CAD build for the part. Positions are in the model's coordinates, mm. Face numbers are marked on the shaded views. Round coordinates to 2 decimals unless told otherwise and drop trailing zeros. Order: outer loops, then holes, each group sorted by start corner. A loop starts at its lowest first (then second) coordinate and runs counter-clockwise, first axis right, second up. Notation, with made-up numbers: M -15,11 L 17,11 A17 ccw 17,38 Z; hole C 33,4 d3. An arc over 180 degrees is marked long. Put each result on its own line as item: value.
Autodesk Inventor part; units mm, degrees
ref_plane "YZ Plane" through (0, 0, 0) normal (1, 0, 0) x (0, 1, 0)
ref_plane "XZ Plane" through (0, 0, 0) normal (0, 1, 0) x (-1, 0, 0)
ref_plane "XY Plane" through (0, 0, 0) normal (0, 0, 1) x (1, 0, 0)
sketch "Sketch1" plane through (0, 0, 0) normal (0, 1, 0) x (-1, 0, 0)
  line L0 (0, 0) -> (0, -60) construction
  line L1 (-60, 0) -> (-60, -60)
  line L2 (60, -60) -> (60, 0)
  arc A0 (60, 0) -> (-60, 0) centre (0, 0) ccw
  arc A1 (-60, -60) -> (60, -60) centre (0, -60) ccw
  line L3 (56, 0) -> (56, -60)
  arc A2 (-56, -60) -> (56, -60) centre (0, -60) ccw
  line L4 (-56, -60) -> (-56, 0)
  arc A3 (56, 0) -> (-56, 0) centre (0, 0) ccw
  point P0 (0, -30)
  dimension "d0" = 60
  dimension "d1" = 60
  dimension "d4" = 4
extrude "Extrusion2" add sketch "Sketch1" along normal blind 70
extrude "Extrusion3" add sketch "Sketch1" along normal blind 4 contours L3 A2 L4 A3
fillet "Fillet1" radius 50.8 8 edges at (0, 4, 56) (-56, 4, -30) (0, 4, -116) (56, 4, -30) (0, 0, 60) (60, 0, -30) (0, 0, -120) (-60, 0, -30)
sketch "Sketch5" plane through (0, 70, 0) normal (0, 1, 0) x (1, 0, 0)
  line L0 (-9, 118.645) -> (9, 118.645)
  line L1 (9, 118.645) -> (9, -58.355)
  line L2 (9, -58.355) -> (-9, -58.355)
  line L3 (-9, -58.355) -> (-9, 118.645)
  point P0 (0, 0)
  dimension "d11" = 177
  dimension "d12" = 18
  dimension "d13" = 9
extrude "Extrusion4" add sketch "Sketch5" against normal blind 10
extrude "Extrusion5" cut sketch "Sketch5" against normal blind 9
sketch "Sketch6" plane through (0, 61, 0) normal (0, 1, 0) x (1, 0, 0)
  line L0 (-9, 118.6362) -> (9, 118.6362)
  line L1 (9, 118.6362) -> (9, -58.3638)
  line L2 (9, -58.3638) -> (-9, -58.3638)
  line L3 (-9, -58.3638) -> (-9, 118.6362)
  line L4 (-8, 117.6362) -> (8, 117.6362)
  line L5 (8, 117.6362) -> (8, -57.3638)
  line L6 (8, -57.3638) -> (-8, -57.3638)
  line L7 (-8, -57.3638) -> (-8, 117.6362)
  point P0 (0, 0)
  dimension "d19" = 177
  dimension "d20" = 18
  dimension "d21" = 9
  dimension "d22" = 1
extrude "Extrusion6" add sketch "Sketch6" along normal blind 5.5
properties part number "lid"
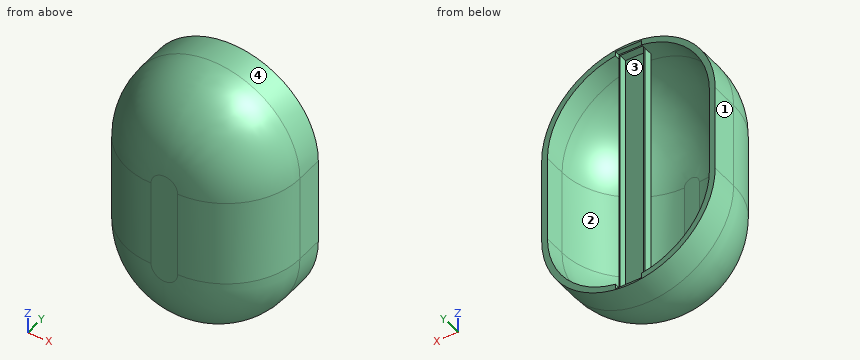
Item 1: Pin check, flat tips, straight feed: P1, Ø5, axis at x = -4.5, z = -33, coming from the +Y side; P2, Ø4.5, axis at y = 63, z = -70, coming from the +X side; P3, Ø2.5, axis at y = 68, z = 56.5, coming from the -X side; P4, Ø3, axis at y = 63, z = -61.5, coming from the -X side. Stop position of each tip, or through.
Answers below:
P1: y = 61
P2: x = 59.5
P3: x = -23.4
P4: x = -60
Item 2: Probe line 1 along Y through (x, z) = (-6.5, -35); line 2 along Z through (x, y) = (-39.5, 27); line 3 along X through (y, z) = (56, -44). List the from-to ranges inside material, lowest first. Write a range as [from, to].
Answers below:
line 1: [0, 4.02], [60, 61]
line 2: [-96.94, -86.77], [26.77, 36.94]
line 3: [-60, -56], [56, 60]
Item 3: Mould opens along Z. For the marked faces 1, 2, 3 and 4 say: pulls with the +Z half, pulls with the -Z half, needs draft (parallel to the pull), parting line crosses it, or undercut.
Answers below:
face 1: needs draft
face 2: undercut
face 3: undercut
face 4: pulls with the +Z half
Item 4: Band-saw the part on A-A on z = -12. Give the cut face in (x, y), and give its area (3 significant figures).
Answers below:
outline: M -60,50.8 A50.8 ccw -9.2,0 L 9.2,0 A50.8 ccw 60,50.8 L 60,70 L 56,70 L 56,54.8 A50.8 cw 5.2,4 L -5.2,4 A50.8 cw -56,54.8 L -56,70 L -60,70 Z; M -9,60 L 9,60 L 9,66.5 L 8,66.5 L 8,61 L -8,61 L -8,66.5 L -9,66.5 Z
area: 1,040 mm²
